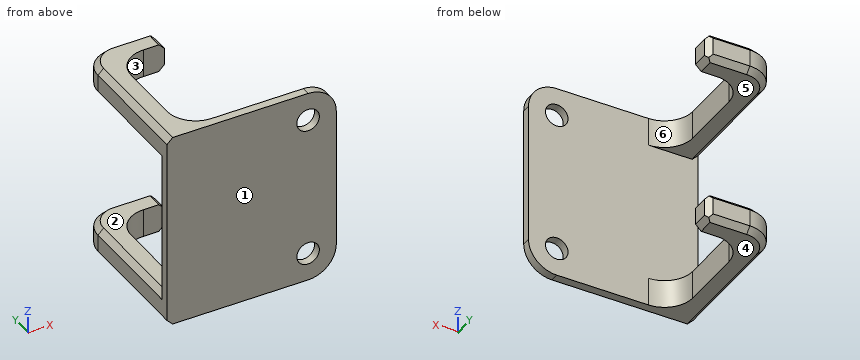
Autodesk Inventor part; units mm, degrees
ref_plane "YZ Plane" through (0, 0, 0) normal (1, 0, 0) x (0, 1, 0)
ref_plane "XZ Plane" through (0, 0, 0) normal (0, 1, 0) x (-1, 0, 0)
ref_plane "XY Plane" through (0, 0, 0) normal (0, 0, 1) x (1, 0, 0)
sketch "Sketch1" plane through (0, 0, 0) normal (0, 0, 1) x (1, 0, 0)
  line L0 (0, 0) -> (0, 50)
  line L1 (0, 50) -> (25, 50)
  line L2 (25, 50) -> (25, 42.5)
  line L3 (25, 42.5) -> (7.5, 42.5)
  line L4 (7.5, 42.5) -> (7.5, 0)
  line L5 (7.5, 0) -> (0, 0)
  line L6 (0, 0) -> (-20, 0)
  line L7 (-20, 0) -> (-20, -3)
  line L8 (-20, -3) -> (60, -3)
  line L9 (60, -3) -> (60, 0)
  line L10 (60, 0) -> (7.5, 0)
  line L11 (0, 0) -> (0, -3)
  dimension "d0" = 50
  dimension "d1" = 25
  dimension "d2" = 7.5
  dimension "d3" = 17.5
  dimension "d4" = 20
  dimension "d5" = 3
  dimension "d6" = 80
extrude "Extrusion1" add sketch "Sketch1" along normal blind 10 contours L5 L10 L9 L8 L11
extrude "Extrusion2" add sketch "Sketch1" along normal blind 10 contours L0 L1 L2 L3 L4 L5
extrude "Extrusion3" add sketch "Sketch1" against normal blind 60 contours L5 L10 L9 L8 L11
extrude "Extrusion4" add sketch "Sketch1" against normal blind 60 contours L0 L1 L2 L3 L4 L5
extrude "Extrusion5" cut sketch "Sketch1" against normal blind 50 contours L0 L1 L2 L3 L4 L5
fillet "Fillet1" radius 10 5 edges at (60, -1.5, 10) (60, -1.5, -60) (7.5, 0, 5) (7.5, 42.5, 5) (7.5, 42.5, -55)
fillet "Fillet2" radius 10 2 edges at (0, 50, -55) (0, 50, 5)
chamfer "Chamfer1" distance 2 angle 45 12 edges at (0, 18.5, -60) (2.9289, 47.0711, -60) (17.5, 50, -60) (0, 18.5, 10) (2.9289, 47.0711, 10) (17.5, 50, 10) (0, 20, -50) (2.9289, 47.0711, -50) (17.5, 50, -50) (0, 20, 0) (2.9289, 47.0711, 0) (17.5, 50, 0)
chamfer "Chamfer2" distance 2 angle 45 6 edges at (25, 45.25, -60) (25, 50, -55) (25, 45.25, -50) (25, 45.25, 0) (25, 45.25, 10) (25, 50, 5)
sketch "Sketch2" plane through (17.5, 0, 10) normal (0, 1, 0) x (1, 0, 0)
  arc A0 (32.5, 0) -> (42.5, 10) centre (32.5, 10) ccw
  arc A1 (42.5, 60) -> (32.5, 70) centre (32.5, 60) ccw
  circle A2 centre (32.5, 10) radius 4
  circle A3 centre (32.5, 60) radius 4
  point P0 (-17.5, 10)
  dimension "d25" = 8
  dimension "d26" = 8
extrude "Extrusion6" cut sketch "Sketch2" against normal blind 60
properties part number "Hook"
Can you work these out from the model? Positions are in its coordinate system, mm. Face numbers are marked on the shaded views. A direction names the side the tool comes from. Coordinates: 2 decimals unless noted, no trailing zeros. Write each loop counter-clockwise with the first axis right and the second up, starting at its lowest first coordinate (ties: lowest second). Pieces come first, ordered by that corner, then holes. Notation, with made-up numbers: (-3, 10.5) - (34, 10.5) arc R20 cw to (34, 36.5) - close; hole circle Ø5 at (78, -26.75). An arc over 180 degrees is marked (long way). Return JSON: item names as keys, results as strings. Group by question number.
Item 1: If we section it at B-B (y = 17): Write out the boundary of the cut face in (x, z), then the cut area to 3 significant figures.
Item 2: If we section it at C-C (z = -11.5): Write out the boundary of the cut face in (x, y).
Item 3: If we section it at D-D (x = 34): Write out the boundary of the cut face in (y, z).
Item 4: If we section it at A-A (x = 20): Write out the boundary of the cut face in (y, z), then the cut area to 3 significant figures.
Item 5: Please list where these lines run through material, in increasing order: probe 1 along Z at (x, y) = (50, -2.3); probe 2 along X at (y, z) = (-0.85, 0); probe 3 along Z at (x, y) = (3.5, 2).
Item 6: I'm going to push flat-ended pins straight in: pin 1 Ø4.5 at (y, z) = (45.5, -55.5) entering from +X; pin 2 Ø8 at (x, z) = (43, 0) entering from +Y; pin 3 Ø6.5 at (x, y) = (13, 32) entering from -Z; pin 4 Ø10 at (y, z) = (26, -51.5) entering from +X. Where does each tip first touch, or does it pass through?
Item 7: We'd pull the mould along Y, two halves only. Please class the marked faces 1, 2 and 3: pulls with the +Y half, pulls with the -Y half, needs draft (parallel to the pull), parting line crosses it, or undercut.
Item 8: Which directions (+Z, -Z, +X, -X, +Y, -Y) give clear straight access to the entire face, cutting with the end or side of a thin tool? Please do the marked faces 4, 5 and 6.
Return value:
{
 "1": {"outline": "(0, -58) - (2, -60) - (7.5, -60) - (7.5, -50) - (2, -50) - (0, -52) - close; (0, 2) - (2, 0) - (7.5, 0) - (7.5, 10) - (2, 10) - (0, 8) - close", "area": "142 mm^2"},
 "2": {"outline": "(0, -3) - (60, -3) - (60, 0) - (0, 0) - close"},
 "3": {"outline": "(-3, -60) - (0, -60) - (0, 10) - (-3, 10) - close"},
 "4": {"outline": "(-3, -60) - (0, -60) - (0, 10) - (-3, 10) - close; (42.5, -60) - (48, -60) - (50, -58) - (50, -52) - (48, -50) - (42.5, -50) - close; (42.5, 0) - (48, 0) - (50, 2) - (50, 8) - (48, 10) - (42.5, 10) - close", "area": "352 mm^2"},
 "5": {"probe 1": "z = -60 to -54, -46 to -4, 4 to 10", "probe 2": "x = 0 to 46, 54 to 60", "probe 3": "z = -60 to -50, 0 to 10"},
 "6": {"pin 1": "stops at x = 25", "pin 2": "stops at y = 0", "pin 3": "passes through", "pin 4": "stops at x = 7.5"},
 "7": {"face 1": "pulls with the -Y half", "face 2": "needs draft", "face 3": "undercut"},
 "8": {"face 4": "-Z, +X, -X, +Y, -Y", "face 5": "+X, -X, +Y", "face 6": "+Z, -Z, +X"}
}
